```python
from build123d import *

# Parameters (mm, degrees)
SKETCH2_W                                    = 160
SKETCH2_H                                    = 80
BOSS_EXTRUDE1_DEPTH                          = 4
SKETCH3_W                                    = 22
SKETCH3_H                                    = 18
CUT_EXTRUDE1_DEPTH                           = 11
CBORE_FOR_M3_HEX_SOCKET_HEAD_CAP_SCR_2_COUNT = 2
CBORE_FOR_M3_HEX_SOCKET_HEAD_CAP_SCR_2_PITCH = 150
CBORE_FOR_M3_HEX_SOCKET_HEAD_CAP_SCR_3_COUNT = 2
CBORE_FOR_M3_HEX_SOCKET_HEAD_CAP_SCR_3_PITCH = 165.529453572
CBORE_FOR_M3_HEX_SOCKET_HEAD_CAP_SCR_4_COUNT = 2
CBORE_FOR_M3_HEX_SOCKET_HEAD_CAP_SCR_4_PITCH = 70


with BuildPart() as part:
    # Sketch2 → Boss-Extrude1 (new body)
    with BuildSketch(Plane(origin=(0, 0, 0), x_dir=(1, 0, 0), z_dir=(0, 1, 0))):
        Rectangle(SKETCH2_W, SKETCH2_H)
    extrude(amount=BOSS_EXTRUDE1_DEPTH)

    # Sketch3 → Cut-Extrude1 (cut)
    with BuildSketch(Plane(origin=(0, 4, 0), x_dir=(1, 0, 0), z_dir=(0, 1, 0))):
        with Locations((-54.553971888, -0.568270541)):
            Rectangle(SKETCH3_W, SKETCH3_H)
        with Locations((53.579793819, -0.081181506)):
            Rectangle(SKETCH3_W, SKETCH3_H)
    extrude(amount=-CUT_EXTRUDE1_DEPTH, mode=Mode.SUBTRACT)

    # Sketch7 → CBORE for M3 Hex Socket Head Cap Screw1 (revolve, cut)
    with BuildSketch(Plane(origin=(-75, 4, -35), x_dir=(0, 0, 1), z_dir=(1, 0, 0))):
        Polygon((0, 0), (0, 4), (1.7, 4), (1.7, 3.4), (3.25, 3.4), (3.25, 0.025), (3.275, 0), align=None)
    cbore_for_m3_hex_socket_head_cap_screw1 = revolve(axis=Axis((-75, 10.35, -35), (0, -1, 0)), mode=Mode.SUBTRACT)

    # CBORE for M3 Hex Socket Head Cap Scr 2: CBORE for M3 Hex Socket Head Cap Screw1 ×2
    with Locations(*[(i * CBORE_FOR_M3_HEX_SOCKET_HEAD_CAP_SCR_2_PITCH, 0, 0) for i in range(1, CBORE_FOR_M3_HEX_SOCKET_HEAD_CAP_SCR_2_COUNT)]):
        add(cbore_for_m3_hex_socket_head_cap_screw1, mode=Mode.SUBTRACT)

    # CBORE for M3 Hex Socket Head Cap Scr 3: CBORE for M3 Hex Socket Head Cap Screw1 ×2
    with Locations(*[Vector(0.9061831399952655, 0, 0.4228854653311239) * (i * CBORE_FOR_M3_HEX_SOCKET_HEAD_CAP_SCR_3_PITCH) for i in range(1, CBORE_FOR_M3_HEX_SOCKET_HEAD_CAP_SCR_3_COUNT)]):
        add(cbore_for_m3_hex_socket_head_cap_screw1, mode=Mode.SUBTRACT)

    # CBORE for M3 Hex Socket Head Cap Scr 4: CBORE for M3 Hex Socket Head Cap Screw1 ×2
    with Locations(*[(0, 0, i * CBORE_FOR_M3_HEX_SOCKET_HEAD_CAP_SCR_4_PITCH) for i in range(1, CBORE_FOR_M3_HEX_SOCKET_HEAD_CAP_SCR_4_COUNT)]):
        add(cbore_for_m3_hex_socket_head_cap_screw1, mode=Mode.SUBTRACT)


solid = part.part
```
Build history of the part. All positions in model axes, mm. A direction names the side the tool comes from. Give positions to 0.01 mm unless a question says otherwise; leave off trailing zeros. Order: outer loops, then holes, each group sorted by start corner. A loop starts at its lowest first (then second) coordinate and runs counter-clockwise, first axis right, second up. Notation, with made-up numbers: M -3.5,57.5 L 2.5,57.5 A4 cw 2.5,62.5 Z; hole C -6,29.5 d8. An arc over 180 degrees is marked long. Write item = value, one per line. Start each with the question number.
(1) Pin check, flat tips, straight feed: pin 1 Ø4 at (x, z) = (-75, -35) entering from -Y; pin 2 Ø6 at (x, z) = (-75, 35) entering from +Y. Stop position of each tip, or through.
(2) Slice it at D-D on z = 4. Write the cut outline in (x, y), plus the area to 3 significant figures.
(3) Slice it at B-B on x = 75. Write the cut outline in (y, z) (3 decimals), plus the area to 3 significant figures.
(4) Which spindle directions (+Z, -Z, +X, -X, +Y, -Y) get a long thin tool onto all of the face, cutting with end or side? Do faces 4 (the flat face through (-1, 2, -40)), 5 (the flat face through (-73.6, 0.6, -36.4)), 6 (the flat face through (64.58, 2, 0)). Say none if no direction does.
(5) Two-plate mould, pull along X, no slides. Class faces 1 (the flat face through (80, 2, 1)), 2 (the flat face through (-1, 0, -1)), 3 (the flat face through (-73.6, 0.6, 33.6)): released by +X, released by -X, zero draft, split by the parting line, or undercut.
(6) Slice it at C-C on y = 1.7. Write the cut outline in (x, z), plus the area to 3 significant figures.
(7) Slice it at A-A on z = -35. Write the cut outline in (x, y) (3 decimals), plus the area to 3 significant figures.
(8) Probe L1, parallel to Z at x = -75, y = 1.65; L2, parallel to Z at x = 75, y = 0.4; L3, parallel to X at y = 0.35, z = -4. List the from-to ranges inside material, lowest first. Write a range as [from, to].
Responses:
q1.pin_1 = 0
q1.pin_2 = 0.6
q2.outline = M -80,0 L -65.55,0 L -65.55,4 L -80,4 Z; M -43.55,0 L 42.58,0 L 42.58,4 L -43.55,4 Z; M 64.58,0 L 80,0 L 80,4 L 64.58,4 Z
q2.area = 464 mm2
q3.outline = M 0,-40 L 4,-40 L 4,-38.275 L 3.975,-38.25 L 0.6,-38.25 L 0.6,-36.7 L 0,-36.7 Z; M 0,-33.3 L 0.6,-33.3 L 0.6,-31.75 L 3.975,-31.75 L 4,-31.725 L 4,31.725 L 3.975,31.75 L 0.6,31.75 L 0.6,33.3 L 0,33.3 Z; M 0,36.7 L 0.6,36.7 L 0.6,38.25 L 3.975,38.25 L 4,38.275 L 4,40 L 0,40 Z
q3.area = 272 mm2
q4.face_4 = -Z, +X, -X, +Y, -Y
q4.face_5 = +Y
q4.face_6 = +Y, -Y
q5.face_1 = released by +X
q5.face_2 = zero draft
q5.face_3 = undercut
q6.outline = M -80,-40 L 80,-40 L 80,40 L -80,40 Z; hole C -75,-35 d6.5; hole C -75,35 d6.5; hole M -65.55,-8.43 L -43.55,-8.43 L -43.55,9.57 L -65.55,9.57 Z; hole M 42.58,-8.92 L 64.58,-8.92 L 64.58,9.08 L 42.58,9.08 Z; hole C 75,-35 d6.5; hole C 75,35 d6.5
q6.area = 11,900 mm2
q7.outline = M -80,0 L -76.7,0 L -76.7,0.6 L -78.25,0.6 L -78.25,3.975 L -78.275,4 L -80,4 Z; M -73.3,0 L 73.3,0 L 73.3,0.6 L 71.75,0.6 L 71.75,3.975 L 71.725,4 L -71.725,4 L -71.75,3.975 L -71.75,0.6 L -73.3,0.6 Z; M 76.7,0 L 80,0 L 80,4 L 78.275,4 L 78.25,3.975 L 78.25,0.6 L 76.7,0.6 Z
q7.area = 592 mm2
q8.L1 = [-40, -38.25], [-31.75, 31.75], [38.25, 40]
q8.L2 = [-40, -36.7], [-33.3, 33.3], [36.7, 40]
q8.L3 = [-80, -65.55], [-43.55, 42.58], [64.58, 80]
